Build history of the part. All positions in model axes, mm. Face numbers are marked on the shaded views. Round coordinates to 2 decimals unless told otherwise and drop trailing zeros. Loops run counter-clockwise (first coordinate to the right, second up) from the corner with the lowest first, then second, coordinate; pieces in that order, holes last. Notation, with made-up numbers: (30, 13.25) - (70, 13.25) arc R33 ccw to (70, 47.25) - close; hole circle Ø11 at (26, 44). An arc over 180 degrees is marked (long way). Use a Markdown table: item, result.
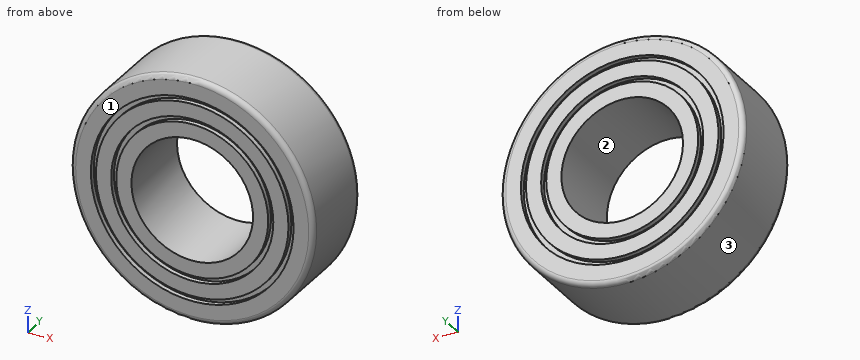
from build123d import *

# Parameters (mm, degrees)
F0_W     = 3
F0_H     = 4
F2_R     = 5
F2_R_2   = 4.75
F2_R_3   = 4
F2_R_4   = 3.75
F3_DEPTH = 0.25
F4_R     = 0.25


# Not quite as in the source:
# - a pattern or mirror of a feature is missing from the dataset's text; its kind, count and spacing are read off the source's solid


with BuildPart() as f1:
    # F0 (on Top) → F1 (revolve)
    with BuildSketch(Plane.XY):
        with Locations((-4.5, 0)):
            Rectangle(F0_W, F0_H)
    revolve(axis=Axis((0, 8.2013355568, 0), (0, 1, 0)))

    # F2 (on face) → F3 (cut)
    with BuildSketch(Plane.XZ.offset(2)):
        Circle(F2_R)
        Circle(F2_R_2, mode=Mode.SUBTRACT)
        Circle(F2_R_3)
        Circle(F2_R_4, mode=Mode.SUBTRACT)
    f3 = extrude(amount=-F3_DEPTH, mode=Mode.SUBTRACT)

    # F3_copies: F3 across plane
    add(f3.mirror(Plane.ZX), mode=Mode.SUBTRACT)

    # F4
    f4_edges = [f1.edges().sort_by_distance(p)[0] for p in [
        (6, -2, 0),
        (6, 2, 0),
    ]]
    fillet(f4_edges, radius=F4_R)


solid = f1.part
Q1. Drop flat-ended pins along their axis: pin 1 (1 mm diameter, centred on x = -3.5, y = 0.5, fed in from +Z); pin 2 (1.5 mm diameter, centred on y = -1.5, z = -2.5, fed in from +X). Give the stop position or say it passes through.
Results found:
| item | result |
|---|---|
| pin 1 | stops at z = 5.2 |
| pin 2 | stops at x = 5.74 |
Q2. Pull direction X, two halves, no side cores. Call the marked faces 1, 2 and 3: pulls with the +X half, pulls with the -X half, needs draft (parallel to the pull), parting line crosses it, or undercut.
Results found:
| item | result |
|---|---|
| face 1 | needs draft |
| face 2 | undercut |
| face 3 | parting line crosses it |
Q3. Cut at A-A, the plane y = -0.3. List the corners of the cut face in (x, z), plus the area to 3 significant figures.
Results found:
| item | result |
|---|---|
| outline | circle Ø12 at (0, 0); hole circle Ø6 at (0, 0) |
| area | 84.8 mm2 |
Q4. Probe line 1 (Z direction, x = 0, y = -0.9); line 2 (Z direction, x = 0, y = -1.85); line 3 (Z direction, x = 0, y = -1.9). List the from-to ranges inside material, lowest first.
Results found:
| item | result |
|---|---|
| line 1 | z = -6 to -3, 3 to 6 |
| line 2 | z = -5.98 to -5, -4.75 to -4, -3.75 to -3, 3 to 3.75, 4 to 4.75, 5 to 5.98 |
| line 3 | z = -5.95 to -5, -4.75 to -4, -3.75 to -3, 3 to 3.75, 4 to 4.75, 5 to 5.95 |
